Job drawing, mm, ordinate dimensions from the low corner. One solid piece. A direction names the side the tool comes from. Coordinates: 2 decimals unless noted, no trailing zeros. Order: outer loops, then holes, each group sorted by start corner. A loop starts at its lowest first (then second) coordinate and runs counter-clockwise, first axis right, second up. Notation, with made-up numbers: (14, 0) - (70, 0) arc R25 cw to (70, 26) - close; hole circle Ø8 at (-36, -16). An arc over 180 degrees is marked (long way). Use a Markdown table: item, result. Add a question column.
1) Two-plate mould, pull along X, no slides. Class the marked faces 3, 4 and 5: +X half, -X half, draft (parallel to the pull), parting line (faces both ways), or undercut.
2) Saw through at C-C on z = 6.5. List the corners of the cut face in (x, y), then the cut area to 3 significant figures.
3) Saw through at A-A on y = 5. List the corners of the cut face in (x, z), then the cut area to 3 significant figures.
4) Drop flat-ended pins along their axis: P1, Ø3, axis at y = 8.5, z = 6.5, coming from the -X side; P2, Ø3, axis at y = 9, z = 11, coming from the -X side. Give the stop position or say it passes through.
5) Tool access for the marked faces 1 and 2: list every direction of +Z, -Z, +X, -X, +Y, -Y with a clear straight run to the whole face (end or side of a thin tool).
6) Saw through at B-B on x = 18. List the corners of the cut face in (y, z), then the cut area to 3 significant figures.
7) Wall check: L1, parallel to Z at x = 17.75, y = 5; L2, parallel to Z at x = 8, y = 2; L3, parallel to X at y = 8.75, z = 6.75. Give the ranges that are in metal, low to high. Write a range as [from, to].
8) Saw through at D-D on z = 12. List the corners of the cut face in (x, y).
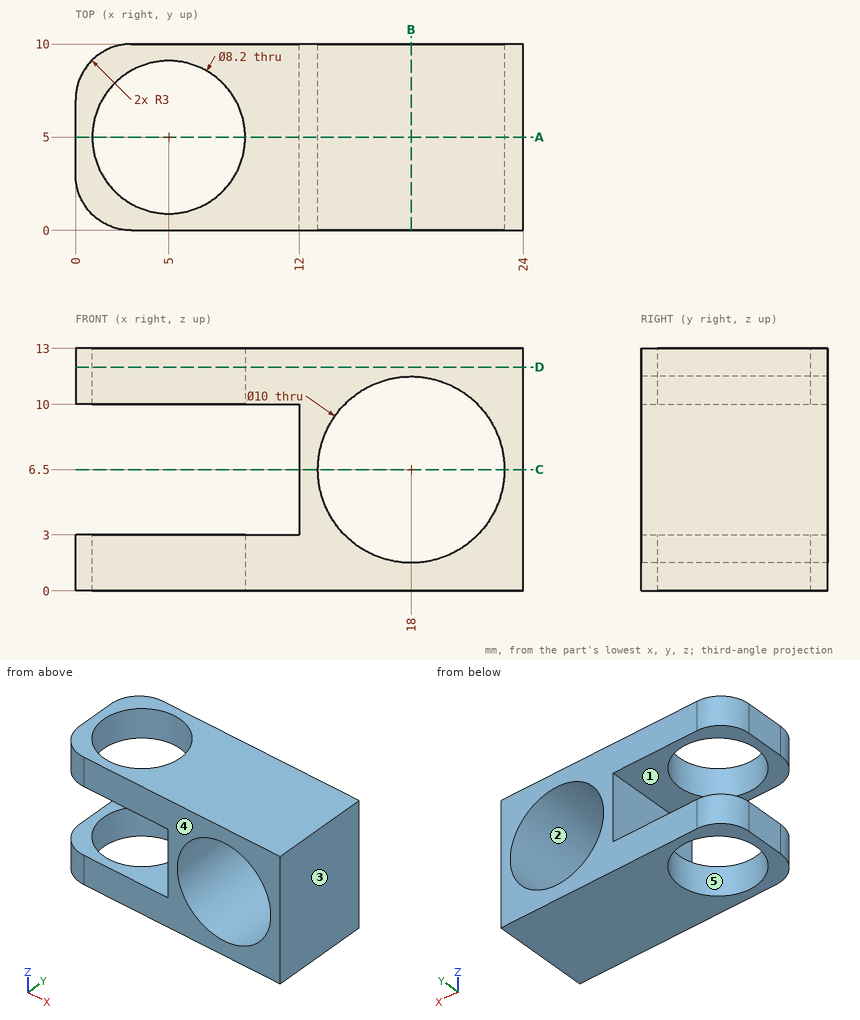
Results are:
| question | item | result |
|---|---|---|
| 1 | face 3 | +X half |
| 1 | face 4 | draft |
| 1 | face 5 | undercut |
| 2 | outline | (12, 0) - (13, 0) - (13, 10) - (12, 10) - close; (23, 0) - (24, 0) - (24, 10) - (23, 10) - close |
| 2 | area | 20.0 mm2 |
| 3 | outline | (0, 0) - (0.9, 0) - (0.9, 3) - (0, 3) - close; (0, 10) - (0.9, 10) - (0.9, 13) - (0, 13) - close; (9.1, 0) - (24, 0) - (24, 13) - (9.1, 13) - (9.1, 10) - (12, 10) - (12, 3) - (9.1, 3) - close; hole circle Ø10 at (18, 6.5) |
| 3 | area | 100 mm2 |
| 4 | P1 | x = 12 |
| 4 | P2 | x = 0.04 |
| 5 | face 1 | -X, +Y, -Y |
| 5 | face 2 | +Y, -Y |
| 6 | outline | (0, 0) - (10, 0) - (10, 1.5) - (0, 1.5) - close; (0, 11.5) - (10, 11.5) - (10, 13) - (0, 13) - close |
| 6 | area | 30.0 mm2 |
| 7 | L1 | [0, 1.51], [11.49, 13] |
| 7 | L2 | [0, 3], [10, 13] |
| 7 | L3 | [12, 13.01], [22.99, 24] |
| 8 | outline | (0, 3) arc R3 ccw to (3, 0) - (24, 0) - (24, 10) - (3, 10) arc R3 ccw to (0, 7) - close; hole circle Ø8.2 at (5, 5) |
